Design review of the part built by this model. Coordinates are the model's own, in mm. Coordinates: 2 decimals unless noted, no trailing zeros. Write each loop counter-clockwise with the first axis right and the second up, starting at its lowest first coordinate (ties: lowest second). Pieces come first, ordered by that corner, then holes. Notation, with made-up numbers: (33, 60) - (67, 60) arc R33 cw to (67, 95) - close; hole circle Ø1 at (85.25, 88). An arc over 180 degrees is marked (long way). One line per item, written item: value.
from build123d import *

# Parameters (mm, degrees)
SKETCH2_W              = 200
SKETCH2_H              = 200
BOSS_EXTRUDE1_DEPTH    = 5
SKETCH3_W              = 5
SKETCH3_H              = 30
BOSS_EXTRUDE2_DEPTH    = 60
CUT_EXTRUDE1_REACH     = 189.75
SKETCH4_R              = 5
FILLET1_R              = 10
LPATTERN1_COUNT        = 3
LPATTERN1_PITCH        = 57.5
LPATTERN1_COUNT_DIR2   = 2
LPATTERN1_PITCH_DIR2   = 136.25
FILLET1_OF_LPATTERN1_R = 10
SKETCH6_R              = 20
CUT_EXTRUDE3_DEPTH     = 154.622914957
SKETCH10_R             = 2.5
CUT_EXTRUDE4_DEPTH     = 154.622914957
LPATTERN2_COUNT        = 3
LPATTERN2_PITCH        = 65
LPATTERN2_COUNT_DIR2   = 2
LPATTERN2_PITCH_DIR2   = 162.5
SKETCH11_W             = 200
SKETCH11_H             = 200
CUT_EXTRUDE5_DEPTH     = 154.622914957
SKETCH12_R             = 7.5
CUT_EXTRUDE6_DEPTH     = 142.509716981


with BuildPart() as part:
    # Sketch2 → Boss-Extrude1 (new body)
    with BuildSketch(Plane(origin=(0, 0, 0), x_dir=(1, 0, 0), z_dir=(0, 1, 0))):
        Rectangle(SKETCH2_W, SKETCH2_H)
    extrude(amount=BOSS_EXTRUDE1_DEPTH)

    # Sketch3 → Boss-Extrude2 (add)
    with BuildSketch(Plane(origin=(0, 5, 0), x_dir=(1, 0, 0), z_dir=(0, 1, 0))):
        with Locations((-82.5, 81.25)):
            Rectangle(SKETCH3_W, SKETCH3_H)
        with Locations((-47.5, 81.25)):
            Rectangle(SKETCH3_W, SKETCH3_H)
    boss_extrude2 = extrude(amount=BOSS_EXTRUDE2_DEPTH)

    # Cut-Extrude1: up to this face of the body (flat: up to its plane)
    cut_extrude1_end = Plane(part.part.faces().sort_by_distance((-85, 35, -81.25))[0])
    # Sketch4 → Cut-Extrude1 (cut, up to the picked face)
    with BuildSketch(Plane(origin=(-45, 0, 0), x_dir=(0, 0, -1), z_dir=(1, 0, 0)), mode=Mode.PRIVATE) as cut_extrude1_sk1:
        with Locations((81.25, 55)):
            Circle(SKETCH4_R)
    cut_extrude1_tool1 = split(extrude(cut_extrude1_sk1.sketch, amount=-CUT_EXTRUDE1_REACH, mode=Mode.PRIVATE), bisect_by=cut_extrude1_end, keep=Keep.BOTH, mode=Mode.PRIVATE)
    cut_extrude1 = cut_extrude1_tool1.solids().sort_by(Axis((-45, 55, -81.25), (-1, 0, 0)))[0]
    add(cut_extrude1, mode=Mode.SUBTRACT)

    # Fillet1
    fillet1_edges = [part.edges().sort_by_distance(p)[0] for p in [
        (-82.5, 65, -96.25),
        (-82.5, 65, -66.25),
        (-47.5, 65, -96.25),
        (-47.5, 65, -66.25),
    ]]
    fillet(fillet1_edges, radius=FILLET1_R)

    # LPattern1: Boss-Extrude2, Cut-Extrude1 3 × 2
    with Locations(*[(i * LPATTERN1_PITCH, 0, j * LPATTERN1_PITCH_DIR2) for i in range(LPATTERN1_COUNT) for j in range(LPATTERN1_COUNT_DIR2) if (i, j) != (0, 0)]):
        add(boss_extrude2)
        add(cut_extrude1, mode=Mode.SUBTRACT)

    # Fillet1 of LPattern1
    fillet1_of_lpattern1_edges = [part.edges().sort_by_distance(p)[0] for p in [
        (-82.5, 65, 40),
        (-82.5, 65, 70),
        (-47.5, 65, 40),
        (-47.5, 65, 70),
        (-25, 65, -96.25),
        (-25, 65, -66.25),
        (10, 65, -96.25),
        (10, 65, -66.25),
        (-25, 65, 40),
        (-25, 65, 70),
        (10, 65, 40),
        (10, 65, 70),
        (32.5, 65, -96.25),
        (32.5, 65, -66.25),
        (67.5, 65, -96.25),
        (67.5, 65, -66.25),
        (32.5, 65, 40),
        (32.5, 65, 70),
        (67.5, 65, 40),
        (67.5, 65, 70),
    ]]
    fillet(fillet1_of_lpattern1_edges, radius=FILLET1_OF_LPATTERN1_R)

    # Sketch6 → Cut-Extrude3 (cut, through all)
    with BuildSketch(Plane(origin=(0, 5, 0), x_dir=(1, 0, 0), z_dir=(0, 1, 0))):
        with Locations(Location((0, 0, 0), (0, 0, 270))):
            Circle(SKETCH6_R)
    extrude(amount=-CUT_EXTRUDE3_DEPTH, mode=Mode.SUBTRACT)

    # Sketch10 → Cut-Extrude4 (cut, through all)
    with BuildSketch(Plane(origin=(0, 5, 0), x_dir=(1, 0, 0), z_dir=(0, 1, 0))):
        with Locations(Location((-65, 88.75, 0), (0, 0, 270))):
            Circle(SKETCH10_R)
        with Locations(Location((-65, 73.75, 0), (0, 0, 270))):
            Circle(SKETCH10_R)
    cut_extrude4 = extrude(amount=-CUT_EXTRUDE4_DEPTH, mode=Mode.SUBTRACT)

    # LPattern2: Cut-Extrude4 3 × 2
    with Locations(*[(i * LPATTERN2_PITCH, 0, j * LPATTERN2_PITCH_DIR2) for i in range(LPATTERN2_COUNT) for j in range(LPATTERN2_COUNT_DIR2) if (i, j) != (0, 0)]):
        add(cut_extrude4, mode=Mode.SUBTRACT)

    # Sketch11 → Cut-Extrude5 (cut, through all)
    with BuildSketch(Plane(origin=(0, 5, 0), x_dir=(1, 0, 0), z_dir=(0, 1, 0))):
        Rectangle(SKETCH11_W, SKETCH11_H)
    extrude(amount=CUT_EXTRUDE5_DEPTH, mode=Mode.SUBTRACT)

    # Sketch12 → Cut-Extrude6 (cut, through all)
    with BuildSketch(Plane(origin=(0, 5, 0), x_dir=(1, 0, 0), z_dir=(0, 1, 0))):
        with Locations(Location((-27.889795318, 49.001974117, 0), (0, 0, 270))):
            Circle(SKETCH12_R)
        with Locations(Location((-48.500694077, -29.961353007, 0), (0, 0, 270))):
            Circle(SKETCH12_R)
        with Locations(Location((38.23257582, -41.020077289, 0), (0, 0, 270))):
            Circle(SKETCH12_R)
        with Locations(Location((52.382098498, 43.433800873, 0), (0, 0, 270))):
            Circle(SKETCH12_R)
    extrude(amount=-CUT_EXTRUDE6_DEPTH, mode=Mode.SUBTRACT)


solid = part.part
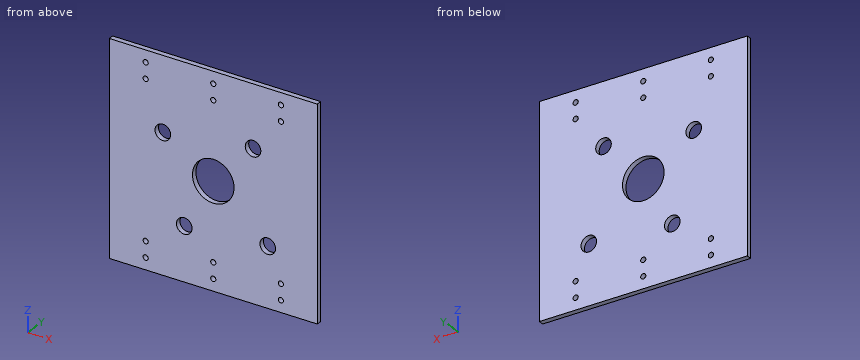
1. Consider section C-C, the plane z = -73.75. Write out the cut boundary in (x, y).
Answer block:
outline: (-100, 0) - (-67.5, 0) - (-67.5, 5) - (-100, 5) - close; (-62.5, 0) - (-2.5, 0) - (-2.5, 5) - (-62.5, 5) - close; (2.5, 0) - (62.5, 0) - (62.5, 5) - (2.5, 5) - close; (67.5, 0) - (100, 0) - (100, 5) - (67.5, 5) - close
2. Consider section B-B, the plane x = 65. Write out the cut boundary in (y, z).
Answer block:
outline: (0, -100) - (5, -100) - (5, -91.25) - (0, -91.25) - close; (0, -86.25) - (5, -86.25) - (5, -76.25) - (0, -76.25) - close; (0, -71.25) - (5, -71.25) - (5, 71.25) - (0, 71.25) - close; (0, 76.25) - (5, 76.25) - (5, 86.25) - (0, 86.25) - close; (0, 91.25) - (5, 91.25) - (5, 100) - (0, 100) - close
3. Wall thickness on line 1 along X through (y, z) = (2.15, 73.75); line 2 along X through (y, z) = (1.35, 74.5); line 3 along Z through (x, y) = (67, 1.3): over which ranges is each line inside the solid? List them lowest first.
Answer block:
line 1: x = -100 to -67.5, -62.5 to -2.5, 2.5 to 62.5, 67.5 to 100
line 2: x = -100 to -67.38, -62.62 to -2.38, 2.38 to 62.62, 67.38 to 100
line 3: z = -100 to -90.25, -87.25 to -75.25, -72.25 to 72.25, 75.25 to 87.25, 90.25 to 100
4. Consider section D-D, the plane x = 0. Write out the cut boundary in (y, z).
Answer block:
outline: (0, -100) - (5, -100) - (5, -91.25) - (0, -91.25) - close; (0, -86.25) - (5, -86.25) - (5, -76.25) - (0, -76.25) - close; (0, -71.25) - (5, -71.25) - (5, -20) - (0, -20) - close; (0, 20) - (5, 20) - (5, 71.25) - (0, 71.25) - close; (0, 76.25) - (5, 76.25) - (5, 86.25) - (0, 86.25) - close; (0, 91.25) - (5, 91.25) - (5, 100) - (0, 100) - close
5. Consider section A-A, the plane z = 0. Write out the cut boundary in (x, y).
Answer block:
outline: (-100, 0) - (-20, 0) - (-20, 5) - (-100, 5) - close; (20, 0) - (100, 0) - (100, 5) - (20, 5) - close
